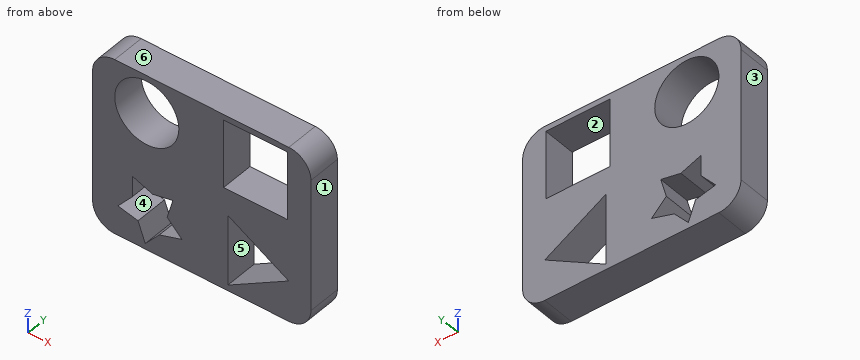
```python
from build123d import *

# Parameters (mm, degrees)
F0_R     = 7.366
F1_DEPTH = 7.62


with BuildPart() as f1:
    # F0 (on Front) → F1 (new body)
    with BuildSketch(Plane.XZ):
        with BuildLine():
            ThreePointArc((0, 5.08), (1.487898, 1.487898), (5.08, 0))
            Line((5.08, 0), (12.3952, 0))
            Line((12.3952, 0), (45.085, 0))
            ThreePointArc((45.085, 0), (48.677102, 1.487898), (50.165, 5.08))
            Line((50.165, 5.08), (50.165, 35.306))
            ThreePointArc((50.165, 35.306), (48.677102, 38.898102), (45.085, 40.386))
            Line((45.085, 40.386), (5.08, 40.386))
            ThreePointArc((5.08, 40.386), (1.487898, 38.898102), (0, 35.306))
            Line((0, 35.306), (0, 5.08))
        make_face()
        Polygon((15.317026, 4.921452), (12.092736, 1.27), (10.433039, 5.720394), (5.811439, 6.816485), (9.150001, 10.650024), (9.150001, 15.391108), (13.79747, 13.581598), (18.444939, 14.500056), (17.134047, 9.934734), (20.529886, 6.519335), align=None, mode=Mode.SUBTRACT)
        Polygon((45.085, 9.3726), (31.050885, 1.27), (31.050885, 17.4752), align=None, mode=Mode.SUBTRACT)
        with Locations((12.446, 31.744603)):
            Circle(F0_R, mode=Mode.SUBTRACT)
        Polygon((30.100089, 39.116), (44.832089, 39.116), (44.832089, 23.538094), (44.832089, 23.451079), (30.100089, 23.451079), align=None, mode=Mode.SUBTRACT)
    extrude(amount=F1_DEPTH)


solid = f1.part
```
Verification items for the finished model (mm, model axes). Face numbers are marked on the shaded views. A direction names the side the tool comes from. Coordinates: 2 decimals unless noted, no trailing zeros. Loops run counter-clockwise (first coordinate to the right, second up) from the corner with the lowest first, then second, coordinate; pieces in that order, holes last. Notation, with made-up numbers: (39, 47.25) -> (70, 47.25) arc R22 cw to (70, 55.25) -> close; hole circle Ø4 at (77, 67). An arc over 180 degrees is marked (long way). Put each result on its own line as item: value.
1. Section check C-C, the plane y = -2. Record the boundary of the cut face in (x, z) (3 decimals).
Result set:
outline: (0, 5.08) arc R5.08 ccw to (5.08, 0) -> (45.085, 0) arc R5.08 ccw to (50.165, 5.08) -> (50.165, 35.306) arc R5.08 ccw to (45.085, 40.386) -> (5.08, 40.386) arc R5.08 ccw to (0, 35.306) -> close; hole circle Ø14.732 at (12.446, 31.745); hole (5.811, 6.816) -> (10.433, 5.72) -> (12.093, 1.27) -> (15.317, 4.921) -> (20.53, 6.519) -> (17.134, 9.935) -> (18.445, 14.5) -> (13.797, 13.582) -> (9.15, 15.391) -> (9.15, 10.65) -> close; hole (30.1, 23.451) -> (44.832, 23.451) -> (44.832, 39.116) -> (30.1, 39.116) -> close; hole (31.051, 1.27) -> (45.085, 9.373) -> (31.051, 17.475) -> close
2. Tool access check on the marked faces 5 and 6. Record the directions out of +Z, -Z, +X, -X, +Y, -Y that give a thin tool (end or side, any length) a straight path to the whole face; none if there is none.
Result set:
face 5: +Y, -Y
face 6: +Z, +X, -X, +Y, -Y
3. Section check A-A, the plane x = 37. Record the boundary of the cut face in (y, z), then the cut area to 3 significant figures.
Result set:
outline: (-7.62, 0) -> (0, 0) -> (0, 4.7) -> (-7.62, 4.7) -> close; (-7.62, 14.04) -> (0, 14.04) -> (0, 23.45) -> (-7.62, 23.45) -> close; (-7.62, 39.12) -> (0, 39.12) -> (0, 40.39) -> (-7.62, 40.39) -> close
area: 117 mm^2
4. Thickness scan on line 1 (X direction, y = -7.25, z = 38.5); line 2 (X direction, y = -2.5, z = 9.5) (3 decimals); line 3 (Z direction, x = 38.5, y = -2). Record the ranges inside material, lowest first.
Result set:
line 1: x = 1.13 to 9.51, 15.38 to 30.1, 44.83 to 49.04
line 2: x = 0 to 8.148, 17.566 to 31.051, 44.864 to 50.165
line 3: z = 0 to 5.57, 13.17 to 23.45, 39.12 to 40.39
5. Mould release check, pull along X, two halves, no side actions. Record for the marked faces 1, 2, 3 and 4: pulls with the +X half, pulls with the -X half, needs draft (parallel to the pull), parting line crosses it, or undercut.
Result set:
face 1: pulls with the +X half
face 2: undercut
face 3: pulls with the -X half
face 4: undercut
6. Section check B-B, the plane z = 26. Record the boundary of the cut face in (x, y) (3 decimals), then the cut area to 3 significant figures.
Result set:
outline: (0, -7.62) -> (7.835, -7.62) -> (7.835, 0) -> (0, 0) -> close; (17.057, -7.62) -> (30.1, -7.62) -> (30.1, 0) -> (17.057, 0) -> close; (44.832, -7.62) -> (50.165, -7.62) -> (50.165, 0) -> (44.832, 0) -> close
area: 200 mm^2
7. Section check D-D, the plane x = 47.5. Record the boundary of the cut face in (y, z), then the cut area to 3 significant figures.
Result set:
outline: (-7.62, 0.61) -> (0, 0.61) -> (0, 39.78) -> (-7.62, 39.78) -> close
area: 298 mm^2
